from build123d import *

# Parameters (mm, degrees)
F0_W     = 90
F0_H     = 46
F1_DEPTH = 3
F3_START = -4.5
F2_W     = 42
F2_H     = 42
F3_DEPTH = 1.5
F4_DEPTH = 1.5


with BuildPart() as f1:
    # F0 (on Right) → F1 (new body, symmetric)
    with BuildSketch(Plane.YZ):
        Rectangle(F0_W, F0_H)
    extrude(amount=F1_DEPTH, both=True)

    # F2 (on face) → F3 (cut)
    with BuildSketch(Plane.YZ.offset(3).offset(F3_START)):
        with Locations((-22, 0)):
            Rectangle(F2_W, F2_H)
        with Locations((22, 0)):
            Rectangle(F2_W, F2_H)
    extrude(amount=-F3_DEPTH, mode=Mode.SUBTRACT)

    # F2 (on face) → F4 (cut)
    with BuildSketch(Plane.YZ.offset(3)):
        with Locations((-22, 0)):
            Rectangle(F2_W, F2_H)
        with Locations((22, 0)):
            Rectangle(F2_W, F2_H)
    extrude(amount=-F4_DEPTH, mode=Mode.SUBTRACT)


solid = f1.part
CAD build for the part. Positions are in the model's coordinates, mm. A direction names the side the tool comes from. Give positions to 0.01 mm unless a question says otherwise; leave off trailing zeros. Write each loop counter-clockwise with the first axis right and the second up, starting at its lowest first coordinate (ties: lowest second). Pieces come first, ordered by that corner, then holes. Notation, with made-up numbers: (7, 73.25) - (63, 73.25) arc R19 ccw to (63, 96.25) - close; hole circle Ø10 at (20, 27.5). An arc over 180 degrees is marked (long way). Answer as CSV lines item,"result".
Q1. Drill centre lines: line 1 (Y direction, x = 2.05, z = 13.5); line 2 (Z direction, x = -2.6, y = 1.5); line 3 (X direction, y = -40, z = 18.5). Where is each one in solid material? Low to high. Write a range as from..to.
Result set:
line 1,"-45..-43, -1..1, 43..45"
line 2,"-23..-21, 21..23"
line 3,"-1.5..1.5"
Q2. Band-saw the part on B-B (z = -16.5). Give the cut face in (x, y).
Result set:
outline,"(-3, -45) - (3, -45) - (3, -43) - (1.5, -43) - (1.5, -1) - (3, -1) - (3, 1) - (1.5, 1) - (1.5, 43) - (3, 43) - (3, 45) - (-3, 45) - (-3, 43) - (-1.5, 43) - (-1.5, 1) - (-3, 1) - (-3, -1) - (-1.5, -1) - (-1.5, -43) - (-3, -43) - close"
Q3. Band-saw the part on A-A (y = -30). Give the cut face in (x, z), and give its area (3 significant figures).
Result set:
outline,"(-3, -23) - (3, -23) - (3, -21) - (1.5, -21) - (1.5, 21) - (3, 21) - (3, 23) - (-3, 23) - (-3, 21) - (-1.5, 21) - (-1.5, -21) - (-3, -21) - close"
area,"150 mm²"
Q4. 3-axis set-ups, long thin cutter, end or side, ignore diameter. For faces 5 (the face through (0, 45, 0)), 6 (the face through (-1.5, -22, 0)): which of +Z, -Z, +X, -X, +Y, -Y reach the whole face in a straight line?
Result set:
face 5,"+Z, -Z, +X, -X, +Y"
face 6,"-X"
Q5. Pull direction Y, two halves, no side cores. Call faces 1 (the face through (0, -1, 23)), 2 (the face through (1.5, 22, 0)), 3 (the face through (0, -45, 0)), 4 (the face through (1.5, -22, 0)): released by +Y, released by -Y, zero draft, split by the parting line, or undercut.
Result set:
face 1,"zero draft"
face 2,"undercut"
face 3,"released by -Y"
face 4,"undercut"
Q6. Flat gauge pins, fed straight in: pin 1 Ø12.5 at (y, z) = (-27.5, -4.5) entering from +X; pin 2 Ø12 at (y, z) = (18.5, 4.5) entering from -X. Where does each tip first touch, or does it go through?
Result set:
pin 1,"x = 1.5"
pin 2,"x = -1.5"
